```python
from build123d import *

# Parameters (mm, degrees)
F0_R     = 6
F1_DEPTH = 25
F3_D     = 5


with BuildPart() as f1:
    # F0 (on Top) → F1 (new body)
    with BuildSketch(Plane.XY):
        with BuildLine():
            Line((-9.069179, 5), (-29, 5))
            Line((-29, 5), (-29, -5))
            Line((-29, -5), (29, -5))
            Line((29, -5), (29, 5))
            Line((29, 5), (9.069179, 5))
            ThreePointArc((9.069179, 5), (5.337433, 7.559835), (6.382015, 11.962963))
            ThreePointArc((6.382015, 11.962963), (0, 28.5), (-6.382015, 11.962963))
            ThreePointArc((-6.382015, 11.962963), (-5.337433, 7.559835), (-9.069179, 5))
        make_face()
        with Locations((0, 19)):
            Circle(F0_R, mode=Mode.SUBTRACT)
    extrude(amount=F1_DEPTH)

    # F3 (through all)
    with Locations(Plane.XZ.offset(5)):
        with Locations((-17.5, 12.5), (17.5, 12.5)):
            Hole(F3_D / 2)


solid = f1.part
```
Here's how the part is built. I have some questions about the finished solid (model axes, mm). Give positions to 0.01 mm unless a question says otherwise; leave off trailing zeros. Loops run counter-clockwise (first coordinate to the right, second up) from the corner with the lowest first, then second, coordinate; pieces in that order, holes last. Notation, with made-up numbers: M 22.25,-13 L 76.25,-13 A26 ccw 76.25,9 Z; hole C 24,55 d6. An arc over 180 degrees is marked long. Put each result on its own line as item: value. Start each with the question number.
(1) I want a section at D-D on y = -1.5. Please give me the cut outline in (x, z), then the cut area to 3 significant figures.
(2) I need wall thicknesses on line 1 along Y through (x, z) = (0, 13); line 2 along Z through (x, y) = (17.5, 0); line 3 along Y through (x, z) = (4, 17.75). Which ranges of each line are inside material? Lowest first, please. Write a range as [from, to].
(3) I want a section at A-A on x = 0. Please give me the cut outline in (y, z).
(4) I want a section at B-B on y = 19. Please give me the cut outline in (x, z).
(5) Will these pins go through, and if not, where does the flat tip stop? pin 1 Ø10 at (x, z) = (-18, 17.5) entering from +Y; pin 2 Ø1 at (y, z) = (10, 3.5) entering from +X; pin 3 Ø2 at (y, z) = (8, 14) entering from -X.
(6) I want a section at C-C on z = 12.5. Please give me the cut outline in (x, y), then the cut area to 3 significant figures.
(7) If we mould it in two halves opening along X, with no side actions, what happens to faces 1 (the flat face through (29, 0, 12)), 2 (the cylindrical face through (19.5, 0.1, 11)), 3 (the flat face through (21, 5, 12))? For each: +X half, -X half, draft (parallel to the pull), parting line (faces both ways), or undercut.
Answer block:
1. outline: M -29,0 L 29,0 L 29,25 L -29,25 Z; hole C -17.5,12.5 d5; hole C 17.5,12.5 d5
1. area: 1,410 mm^2
2. line 1: [-5, 13], [25, 28.5]
2. line 2: [0, 10], [15, 25]
2. line 3: [-5, 14.53], [23.47, 27.62]
3. outline: M -5,0 L 13,0 L 13,25 L -5,25 Z; M 25,0 L 28.5,0 L 28.5,25 L 25,25 Z
4. outline: M -9.5,0 L -6,0 L -6,25 L -9.5,25 Z; M 6,0 L 9.5,0 L 9.5,25 L 6,25 Z
5. pin 1: y = 5
5. pin 2: x = 5.36
5. pin 3: x = -5.61
6. outline: M -29,-5 L -20,-5 L -20,5 L -29,5 Z; M -15,-5 L 15,-5 L 15,5 L 9.07,5 A4 cw 6.38,11.96 A9.5 ccw long -6.38,11.96 A4 cw -9.07,5 L -15,5 Z; M 20,-5 L 29,-5 L 29,5 L 20,5 Z; hole C 0,19 d12
6. area: 709 mm^2
7. face 1: +X half
7. face 2: undercut
7. face 3: draft
